The figure shows three views and two pictorial views of one solid part (mm, origin at its lowest corner). Answer the questions. A direction names the side the tool comes from. Coordinates: 2 decimals unless noted, no trailing zeros. Loops run counter-clockwise (first coordinate to the right, second up) from the corner with the lowest first, then second, coordinate; pieces in that order, holes last. Notation, with made-up numbers: (18.5, 72) -> (29.5, 72) arc R24 ccw to (29.5, 100) -> close; hole circle Ø11 at (47.25, 80). An arc over 180 degrees is marked (long way). Answer in a Markdown table with one row per item.
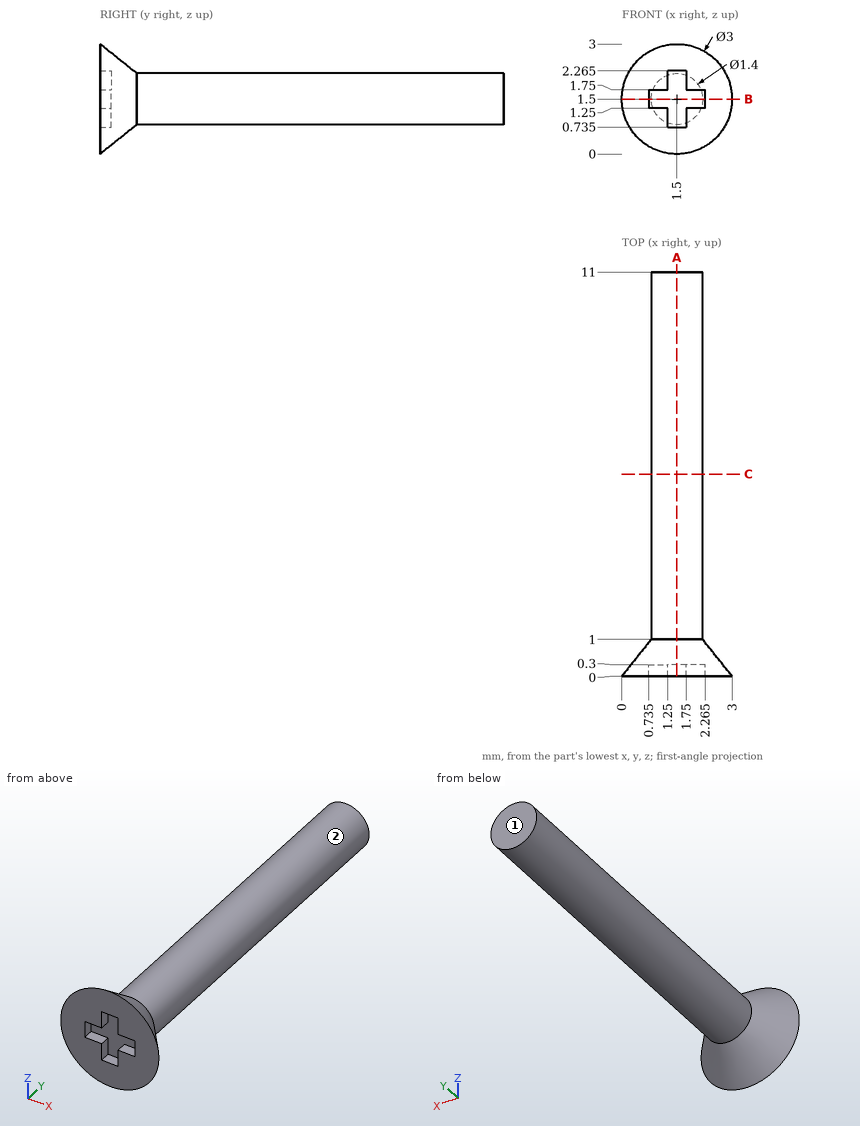
Item 1: A cutting plane is placed at A-A, the plane x = 1.5. Determine the outline of the cut face in (y, z) (3 decimals), plus the area to 3 significant figures.
Findings below:
| item | result |
|---|---|
| outline | (0, 0) -> (1, 0.8) -> (11, 0.8) -> (11, 2.2) -> (1, 2.2) -> (0, 3) -> (0, 2.265) -> (0.3, 2.265) -> (0.3, 0.735) -> (0, 0.735) -> close |
| area | 15.7 mm2 |
Item 2: A cutting plane is placed at B-B, the plane z = 1.5. Determine the outline of the cut face in (x, y) (3 decimals), plus the area to 3 significant figures.
Findings below:
| item | result |
|---|---|
| outline | (0, 0) -> (0.735, 0) -> (0.735, 0.3) -> (2.265, 0.3) -> (2.265, 0) -> (3, 0) -> (2.2, 1) -> (2.2, 11) -> (0.8, 11) -> (0.8, 1) -> close |
| area | 15.7 mm2 |
Item 3: A tool of negligible diameter and unlimited length cuts with its end or side. For the marked faces 1 and 2, from which of +Z, -Z, +X, -X, +Y, -Y can it reach the whole face along a straight path? Write none if from no direction.
Findings below:
| item | result |
|---|---|
| face 1 | +Z, -Z, +X, -X, +Y |
| face 2 | +Y |
Item 4: Flat-ended cylindrical pins translate along their axes: pin 1 Ø1.5 at (y, z) = (3.5, 1.5) entering from +X; pin 2 Ø1 at (x, y) = (1.5, 6.5) entering from -Z. Find the tip coordinate at first contact, or state that the pin passes through.
Findings below:
| item | result |
|---|---|
| pin 1 | stops at x = 2.2 |
| pin 2 | stops at z = 0.8 |
Item 5: Find the intervals of material crossed by probe 1 along Y at (x, z) = (1.6, 1.6); probe 2 along X at (y, z) = (3.5, 1.5); probe 3 along Z at (x, y) = (1.05, 8.5), in increasing order.
Findings below:
| item | result |
|---|---|
| probe 1 | y = 0.3 to 11 |
| probe 2 | x = 0.8 to 2.2 |
| probe 3 | z = 0.96 to 2.04 |
Item 6: A cutting plane is placed at C-C, the plane y = 5.5. Determine the outline of the cut face in (x, z).
Findings below:
| item | result |
|---|---|
| outline | circle Ø1.4 at (1.5, 1.5) |
